Part print with two shaded views. Sizes in mm from the minimum x, y, z corner. Round coordinates to 2 decimals unless told otherwise and drop trailing zeros. Write each loop counter-clockwise with the first axis right and the second up, starting at its lowest first coordinate (ties: lowest second). Pieces come first, ordered by that corner, then holes. Notation, with made-up numbers: (-11, 69) -> (40, 69) arc R27 ccw to (40, 97) -> close; hole circle Ø8 at (10.5, 73.5). An arc over 180 degrees is marked (long way). Answer in a Markdown table with one row per item. Add a question column.
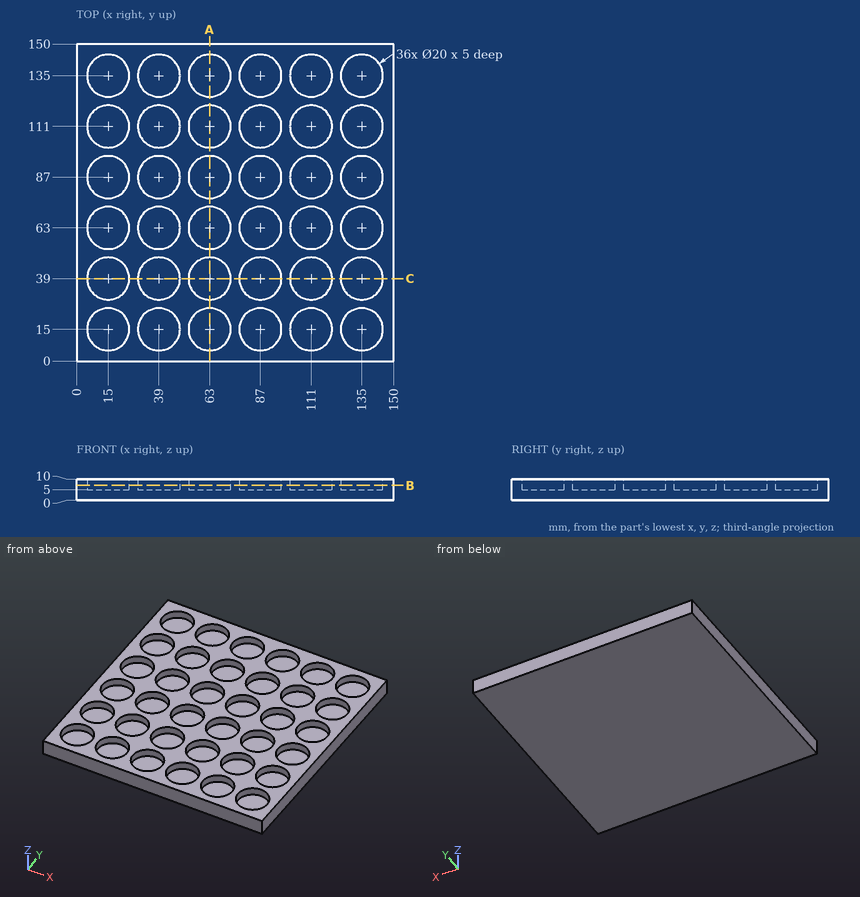
Item 1: Saw through at B-B on z = 7. Count the separate pieces of the cut face and the enclosed holes in it, then the cut area to 3 significant figures.
Item 2: Pin check, flat tip, straight feed: pin 1 (1 mm diameter, centred on x = 92, y = 134, fed in from +Z). Stop position of the tip, or through.
Item 3: Drill centre line: probe 1 along Z at (x, y) = (132, 15). Where is it in solid material? Low to high.
Item 4: Saw through at A-A on x = 63. Give the cut face in (y, z), then the cut area to 3 significant figures.
Recorded:
| question | item | result |
|---|---|---|
| 1 | separate pieces | 1 |
| 1 | enclosed holes | 36 |
| 1 | area | 11,200 mm2 |
| 2 | pin 1 | z = 5 |
| 3 | probe 1 | 0 to 5 |
| 4 | outline | (0, 0) -> (150, 0) -> (150, 10) -> (145, 10) -> (145, 5) -> (125, 5) -> (125, 10) -> (121, 10) -> (121, 5) -> (101, 5) -> (101, 10) -> (97, 10) -> (97, 5) -> (77, 5) -> (77, 10) -> (73, 10) -> (73, 5) -> (53, 5) -> (53, 10) -> (49, 10) -> (49, 5) -> (29, 5) -> (29, 10) -> (25, 10) -> (25, 5) -> (5, 5) -> (5, 10) -> (0, 10) -> close |
| 4 | area | 900 mm2 |
